Work out the finished part from the listing and answer in its coordinate system (mm). A direction names the side the tool comes from. Coordinates: 2 decimals unless noted, no trailing zeros. Order: outer loops, then holes, each group sorted by start corner. A loop starts at its lowest first (then second) coordinate and runs counter-clockwise, first axis right, second up. Notation, with made-up numbers: (-35.75, 49.25) -> (6.25, 49.25) arc R15 ccw to (6.25, 58.25) -> close; hole circle Ø9 at (59.25, 1.5). An arc over 180 degrees is marked (long way). Use one line per item in the form item = value.
from build123d import *

# Parameters (mm, degrees)
F0_R     = 1.5
F1_DEPTH = 5
F2_W     = 15
F2_H     = 15
F3_DEPTH = 25
F4_DEPTH = 20


with BuildPart() as f1:
    # F0 (on Top) → F1 (new body)
    with BuildSketch(Plane.XY):
        Polygon((7.5, -7.5), (7.5, 15), (-7.5, 15), (-7.5, 0), (-7.5, -3.75), (-3.75, -7.5), (0, -7.5), align=None)
        with Locations((-3.75, -3.75)):
            Circle(F0_R, mode=Mode.SUBTRACT)
        with BuildLine():
            Line((7.5, -16.4016504294), (7.5, -7.5))
            Line((7.5, -7.5), (0, -7.5))
            Line((0, -7.5), (-3.75, -7.5))
            ThreePointArc((-3.75, -7.5), (-0.2854517531, -12.6850628714), (-6.4016504294, -13.9016504294))
            Line((-6.4016504294, -13.9016504294), (-6.4016504294, -16.4016504294))
            Line((-6.4016504294, -16.4016504294), (0, -16.4016504294))
            Line((0, -16.4016504294), (7.5, -16.4016504294))
        make_face()
    extrude(amount=F1_DEPTH)

    # F2 (on face) → F3 (cut)
    with BuildSketch(Plane.XY.offset(5)):
        with Locations((0, 7.5)):
            Rectangle(F2_W, F2_H)
    extrude(amount=-F3_DEPTH, mode=Mode.SUBTRACT)

    # F4 (add): a face of the model
    f4_faces = [f1.faces().sort_by_distance(p)[0] for p in [
        (7.5, -8.2008252147, 2.5),
    ]]
    extrude(f4_faces, amount=F4_DEPTH)


solid = f1.part
(1) Section C-C on y = -9.25 is taken. Write down the section's boundary in (x, z), plus the area to 3 significant figures.
Data:
outline = (-0.58, 0) -> (27.5, 0) -> (27.5, 5) -> (-0.58, 5) -> close
area = 140 mm²
(2) Straight lines are drawn through the part: line 1 along Y through (x, z) = (-3.75, 3); line 2 along X through (y, z) = (-11.25, 1.95); line 3 along X through (y, z) = (-14.5, 1.5). For each, find the intervals that lie inside material, in ascending order.
Data:
line_1 = -16.4 to -15, -7.5 to -5.25, -2.25 to 0
line_2 = 0 to 27.5
line_3 = -6.4 to -5.62, -1.88 to 27.5
(3) Section A-A on z = 3.35 is taken. Write down the section's boundary in (x, y), plus the area to 3 significant figures.
Data:
outline = (-7.5, -3.75) -> (-3.75, -7.5) arc R3.75 cw (long way) to (-6.4, -13.9) -> (-6.4, -16.4) -> (27.5, -16.4) -> (27.5, 0) -> (-7.5, 0) -> close; hole circle Ø3 at (-3.75, -3.75)
area = 509 mm²
(4) Which of the six approach directions +Z, -Z, +X, -X, +Y, -Y give full straight-line access (tool end or side, diameter ignored) to faces 1 (the flat face through (10, 0, 3)), 2 (the flat face through (-6.402, -15, 2)), 3 (the flat face through (-5.65, -5.6, 2.46))?
Data:
face_1 = +Z, -Z, +X, -X, +Y
face_2 = +Z, -Z, -X, -Y
face_3 = +Z, -Z, -X
(5) Each of these flat-tipped pins is pushed along its axis until it touches: P1, Ø1.2, axis at y = -15, z = 2, coming from the -X side; P2, Ø6, axis at x = -3.75, y = -11.25, coming from the -Z side; P3, Ø1, axis at y = -12.5, z = 3.5, coming from the -X side. Where does it stop, or does it pass through?
Data:
P1 = -6.4
P2 = through
P3 = -0.43
(6) Section B-B on y = -11.25 is taken. Write down the section's boundary in (x, z).
Data:
outline = (0, 0) -> (27.5, 0) -> (27.5, 5) -> (0, 5) -> close
